```python
from build123d import *

# Parameters (mm, degrees)
SKETCH_1_R      = 15
EXTRUDE_1_DEPTH = 5
EXTRUDE_START   = -25
SKETCH_3_R      = 15
SKETCH_3_R_2    = 10
EXTRUDE_2_DEPTH = 25
FILLET_1_R      = 2


with BuildPart() as part:
    # 草图1 → 凸台-拉伸1 (new body)
    with BuildSketch(Plane(origin=(0, 0, 0), x_dir=(1, 0, 0), z_dir=(0, 1, 0))):
        with Locations(Location((0, 0, 0), (0, 0, 270))):
            Circle(SKETCH_1_R)
    extrude(amount=EXTRUDE_1_DEPTH)

    # 草图3 → 凸台-拉伸2 (add)
    with BuildSketch(Plane(origin=(0, 0, 0), x_dir=(1, 0, 0), z_dir=(0, 1, 0)).offset(EXTRUDE_START)):
        with Locations(Location((0, 0, 0), (0, 0, 270))):
            Circle(SKETCH_3_R)
        with Locations(Location((0, 0, 0), (0, 0, 270))):
            Circle(SKETCH_3_R_2, mode=Mode.SUBTRACT)
    extrude(amount=EXTRUDE_2_DEPTH)

    # 圆角1
    fillet_1_edges = [part.edges().sort_by_distance(p)[0] for p in [
        (0, 5, -15),
    ]]
    fillet(fillet_1_edges, radius=FILLET_1_R)


solid = part.part
```
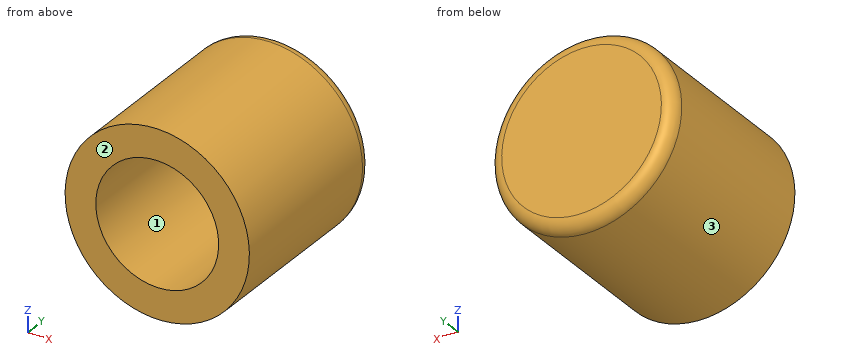
Geometry check sheet. Reference: the model listing, model coordinates, mm. Face numbers are marked on the shaded views. Give positions to 0.01 mm unless a question says otherwise; leave off trailing zeros. Write each loop counter-clockwise with the first axis right and the second up, starting at its lowest first coordinate (ties: lowest second). Pieces come first, ordered by that corner, then holes. Notation, with made-up numbers: (22, 70.5) - (51, 70.5) arc R27 cw to (51, 105.5) - close; hole circle Ø8 at (12.5, 11.5). An arc over 180 degrees is marked (long way). Use a Markdown table: item, result.
Q1. Section check D-D, the plane y = 2.5. Enter the section's corners in (x, z), then the cut area to 3 significant figures.
Computed:
| item | result |
|---|---|
| outline | circle Ø30 at (0, 0) |
| area | 707 mm² |
Q2. Section check A-A, the plane z = 0. Enter the section's corners in (x, y).
Computed:
| item | result |
|---|---|
| outline | (-15, -25) - (-10, -25) - (-10, 0) - (10, 0) - (10, -25) - (15, -25) - (15, 3) arc R2 ccw to (13, 5) - (-13, 5) arc R2 ccw to (-15, 3) - close |
Q3. Section check B-B, the plane x = 0. Enter the section's corners in (y, z).
Computed:
| item | result |
|---|---|
| outline | (-25, -15) - (3, -15) arc R2 ccw to (5, -13) - (5, 13) arc R2 ccw to (3, 15) - (-25, 15) - (-25, 10) - (0, 10) - (0, -10) - (-25, -10) - close |
Q4. Section check C-C, the plane y = -15.75. Enter the section's corners in (x, z).
Computed:
| item | result |
|---|---|
| outline | circle Ø30 at (0, 0); hole circle Ø20 at (0, 0) |
Q5. Thickness scan on L1, parallel to X at y = -6, z = 0; L2, parallel to Z at x = -3, y = -20.75; L3, parallel to Y at x = -4.5, z = 8.25. Record the ranges inside material, lowest first. Write a range as [from, to].
Computed:
| item | result |
|---|---|
| L1 | x = [-15, -10], [10, 15] |
| L2 | z = [-14.7, -9.54], [9.54, 14.7] |
| L3 | y = [0, 5] |
Q6. Draft check along Z on the marked faces 1, 2 and 3. Enter one of: pulls with the +Z half, pulls with the -Z half, needs draft (parallel to the pull), parting line crosses it, or undercut.
Computed:
| item | result |
|---|---|
| face 1 | undercut |
| face 2 | needs draft |
| face 3 | parting line crosses it |
Q7. Go/stop test with flat-tipped pins: P1, Ø6, axis at x = 0, z = 2.5, coming from the -Y side; P2, Ø1, axis at x = 2.5, y = -18.5, coming from the -Z side; P3, Ø6, axis at y = -7, z = 6, coming from the -X side. Record where each tip stops, or that it passes through.
Computed:
| item | result |
|---|---|
| P1 | stops at y = 0 |
| P2 | stops at z = -14.87 |
| P3 | stops at x = -14.7 |
